Read the model definition and answer for the solid it produces. Units are mm, in the model's axes. A direction names the side the tool comes from. Coordinates: 2 decimals unless noted, no trailing zeros. Loops run counter-clockwise (first coordinate to the right, second up) from the corner with the lowest first, then second, coordinate; pieces in that order, holes last. Notation, with made-up numbers: M -5.75,-17 L 22.25,-17 A27 ccw 22.25,-1 Z; hole C 20,9 d6. An arc over 180 degrees is marked long. Use one line per item in the form item = value. Start each with the question number.
1. Find the intervals of material crossed by probe 1 along X at (y, z) = (2.5, -4); probe 2 along Z at (x, y) = (4, 8); probe 3 along Z at (x, y) = (37, 3.5), in increasing order. Write a range as [from, to].
2. The part is cut by section A-A (z = -101). Give the vertices of the cut face in (x, y).
3. A tool of negligible diameter and unlimited length cuts with its end or side. For faces 1 (the flat face through (26, 0, -53)), 2 (the flat face through (34, 7, -97)), 3 (the flat face through (54.5, 2, -48)), from which of +Z, -Z, +X, -X, +Y, -Y can it reach the whole face along a straight path? Write none if from no direction.
4. For a pull along Z with two mould halves and no side action, classify faces 4 (the flat face through (34, 5, -105)), 5 (the cylindrical face through (66.43, 5.58, -4.45)), 6 (the flat face through (4, 11, -49)) as released by +Z, released by -Z, zero draft, split by the parting line, or undercut.
5. The part is cut by section B-B (x = 24). Give the vertices of the cut face in (y, z), plus the area to 3 significant figures.
6. Flat-ended cylindrical pins translate along their axes: pin 1 (5 mm diameter, centred on y = 6.5, z = -30, fed in from +X); pin 2 (2.5 mm diameter, centred on x = 65, z = -4, fed in from -Y); pin 3 (18 mm diameter, centred on x = 35.5, z = -71.5, fed in from +Y); pin 4 (0.9 mm diameter, centred on y = 1.5, z = -67.5, fed in from +X). Find the tip coordinate at first contact, or state that the pin passes through.
7. The part is cut by section C-C (z = -81). Give the vertices of the cut face in (x, y), plus the area to 3 significant figures.
from build123d import *

# Parameters (mm, degrees)
SKETCH1_W           = 69
SKETCH1_H           = 105
BOSS_EXTRUDE2_DEPTH = 11
SKETCH3_W           = 60.642005931
SKETCH3_H           = 87
CUT_EXTRUDE1_DEPTH  = 8
SKETCH4_R           = 1.5
CUT_EXTRUDE2_DEPTH  = 12
SKETCH5_W           = 14.5
SKETCH5_H           = 75
CUT_EXTRUDE3_DEPTH  = 12


with BuildPart() as part:
    # Sketch1 → Boss-Extrude2 (new body)
    with BuildSketch(Plane(origin=(0, 0, 0), x_dir=(1, 0, 0), z_dir=(0, 1, 0))):
        with Locations((34.5, 52.5)):
            Rectangle(SKETCH1_W, SKETCH1_H)
    extrude(amount=BOSS_EXTRUDE2_DEPTH)

    # Sketch3 → Cut-Extrude1 (cut)
    with BuildSketch(Plane(origin=(0, 11, 0), x_dir=(1, 0, 0), z_dir=(0, 1, 0))):
        with Locations((34.678997035, 53.5)):
            Rectangle(SKETCH3_W, SKETCH3_H)
    extrude(amount=-CUT_EXTRUDE1_DEPTH, mode=Mode.SUBTRACT)

    # Sketch4 → Cut-Extrude2 (cut, through all)
    with BuildSketch(Plane(origin=(0, 11, 0), x_dir=(1, 0, 0), z_dir=(0, 1, 0))):
        with Locations((4, 101)):
            Circle(SKETCH4_R)
        with Locations((65, 101)):
            Circle(SKETCH4_R)
        with Locations((4, 4)):
            Circle(SKETCH4_R)
        with Locations((65, 4)):
            Circle(SKETCH4_R)
    extrude(amount=-CUT_EXTRUDE2_DEPTH, mode=Mode.SUBTRACT)

    # Sketch5 → Cut-Extrude3 (cut, through all)
    with BuildSketch(Plane(origin=(0, 11, 0), x_dir=(1, 0, 0), z_dir=(0, 1, 0))):
        with Locations((61.75, 48.9)):
            Rectangle(SKETCH5_W, SKETCH5_H)
    extrude(amount=-CUT_EXTRUDE3_DEPTH, mode=Mode.SUBTRACT)


solid = part.part
Computed values:
q1.probe_1 = [0, 2.5], [5.5, 63.5], [66.5, 69]
q1.probe_2 = [-105, -102.5], [-99.5, -5.5], [-2.5, 0]
q1.probe_3 = [-105, -97], [-10, 0]
q2.outline = M 0,0 L 2.5,0 L 2.5,11 L 0,11 Z; M 5.5,0 L 63.5,0 L 63.5,11 L 5.5,11 Z; M 66.5,0 L 69,0 L 69,11 L 66.5,11 Z
q3.face_1 = +Z, -Z, +X, -X, -Y
q3.face_2 = +Y
q3.face_3 = +X, +Y, -Y
q4.face_4 = released by -Z
q4.face_5 = undercut
q4.face_6 = zero draft
q5.outline = M 0,-105 L 11,-105 L 11,-97 L 3,-97 L 3,-10 L 11,-10 L 11,0 L 0,0 Z
q5.area = 459 mm²
q6.pin_1 = 4.36
q6.pin_2 = through
q6.pin_3 = 3
q6.pin_4 = 54.5
q7.outline = M 0,0 L 54.5,0 L 54.5,3 L 4.36,3 L 4.36,11 L 0,11 Z
q7.area = 198 mm²
